from build123d import *

# Parameters (mm, degrees)
SKETCH_1_R          = 12.95
EXTRUDE_1_DEPTH     = 8
SKETCH_2_R          = 7.05
EXTRUDE_2_DEPTH     = 7
SKETCH_3_R          = 4.25
CUT_EXTRUDE_1_DEPTH = 24.672874773
CHAMFER_1_SIZE      = 0.2


with BuildPart() as part:
    # 草图1 → 凸台-拉伸1 (new body)
    with BuildSketch(Plane(origin=(0, 0, 0), x_dir=(1, 0, 0), z_dir=(0, 1, 0))):
        with Locations(Location((0, 0, 0), (0, 0, 270))):
            Circle(SKETCH_1_R)
    extrude(amount=EXTRUDE_1_DEPTH)

    # 草图2 → 凸台-拉伸2 (add)
    with BuildSketch(Plane(origin=(0, 8, 0), x_dir=(1, 0, 0), z_dir=(0, 1, 0))):
        with Locations(Location((0, 0, 0), (0, 0, 270))):
            Circle(SKETCH_2_R)
    extrude(amount=EXTRUDE_2_DEPTH)

    # 草图3 → 切除-拉伸1 (cut, through all)
    with BuildSketch(Plane.XZ):
        with Locations(Location((0, 0, 0), (0, 0, 270))):
            Circle(SKETCH_3_R)
    extrude(amount=-CUT_EXTRUDE_1_DEPTH, mode=Mode.SUBTRACT)

    # 倒角1
    chamfer_1_edges = [part.edges().sort_by_distance(p)[0] for p in [
        (0, 15, 4.25),
        (0, 0, 4.25),
        (0, 0, -12.95),
        (0, 8, -12.95),
        (0, 15, -7.05),
    ]]
    chamfer(chamfer_1_edges, length=CHAMFER_1_SIZE)


solid = part.part
Work out the finished part from the listing and answer in its coordinate system (mm). A direction names the side the tool comes from. Give positions to 0.01 mm unless a question says otherwise; leave off trailing zeros. Loops run counter-clockwise (first coordinate to the right, second up) from the corner with the lowest first, then second, coordinate; pieces in that order, holes last. Notation, with made-up numbers: (55, -34) - (101, -34) arc R30 cw to (101, -11) - close; hole circle Ø8 at (-18.5, -30.5). An arc over 180 degrees is marked (long way). Answer in a Markdown table with one row per item. Add a question column.
Q1. The part is cut by section A-A (z = 0). Determine the outline of the cut face in (x, y), and give its area (3 significant figures).
Q2. Determine the mould class of faces 3 (the flat face through (-1.4, 15, 4.5)), 4 (the cylindrical face through (-2.7, 11.352, 6.512)), 5 (the cylindrical face through (4.214, 7.398, 0.553)) for opening direction X: released by +X, released by -X, zero draft, split by the parting line, or undercut.
Q3. Consider line 1 along X through (y, z) = (9.75, 0); line 2 along X through (y, z) = (7.5, 0); line 3 along Y through (x, z) = (-6.5, -3). Determine where each line is inside the solid, lowest interval first.
Q4. The part is cut by section B-B (x = 0). Determine the outline of the cut face in (y, z), and give its area (3 significant figures).
Q5. The part is cut by section C-C (y = 14). Determine the outline of the cut face in (x, z), and give its area (3 significant figures).
Q6. The part is cut by section D-D (y = 4.75). Determine the outline of the cut face in (x, z), and give its area (3 significant figures).
Q7. A tool of negligible diameter and unlimited length cuts with its end or side. For faces 1 (the flat face through (-5.5, 8, 5.5)), 2 (the cylindrical face through (3.89, 3.95, 12.35)), from which of +Z, -Z, +X, -X, +Y, -Y can it reach the whole face along a straight path? Write none if from no direction.
Q8. Each of these flat-tipped pins is pushed along its axis until it touches: P1, Ø5, axis at x = 7.5, y = 12, coming from the +Z side; P2, Ø5, axis at y = 13, z = -7.5, coming from the +X side; P3, Ø1.5, axis at x = -8.5, z = -2, coming from the +Y side. Where does it stop, or does it pass through?
Solution:
| question | item | result |
|---|---|---|
| 1 | outline | (-12.95, 0.2) - (-12.75, 0) - (-4.45, 0) - (-4.25, 0.2) - (-4.25, 14.8) - (-4.45, 15) - (-6.85, 15) - (-7.05, 14.8) - (-7.05, 8) - (-12.75, 8) - (-12.95, 7.8) - close; (4.25, 0.2) - (4.45, 0) - (12.75, 0) - (12.95, 0.2) - (12.95, 7.8) - (12.75, 8) - (7.05, 8) - (7.05, 14.8) - (6.85, 15) - (4.45, 15) - (4.25, 14.8) - close |
| 1 | area | 178 mm² |
| 2 | face 3 | zero draft |
| 2 | face 4 | split by the parting line |
| 2 | face 5 | undercut |
| 3 | line 1 | x = -7.05 to -4.25, 4.25 to 7.05 |
| 3 | line 2 | x = -12.95 to -4.25, 4.25 to 12.95 |
| 3 | line 3 | y = 0 to 8 |
| 4 | outline | (0, -12.75) - (0.2, -12.95) - (7.8, -12.95) - (8, -12.75) - (8, -7.05) - (14.8, -7.05) - (15, -6.85) - (15, -4.45) - (14.8, -4.25) - (0.2, -4.25) - (0, -4.45) - close; (0, 4.45) - (0.2, 4.25) - (14.8, 4.25) - (15, 4.45) - (15, 6.85) - (14.8, 7.05) - (8, 7.05) - (8, 12.75) - (7.8, 12.95) - (0.2, 12.95) - (0, 12.75) - close |
| 4 | area | 178 mm² |
| 5 | outline | circle Ø14.1 at (0, 0); hole circle Ø8.5 at (0, 0) |
| 5 | area | 99.4 mm² |
| 6 | outline | circle Ø25.9 at (0, 0); hole circle Ø8.5 at (0, 0) |
| 6 | area | 470 mm² |
| 7 | face 1 | +Y |
| 7 | face 2 | +Y, -Y |
| 8 | P1 | stops at z = 4.97 |
| 8 | P2 | stops at x = 4.97 |
| 8 | P3 | stops at y = 8 |
